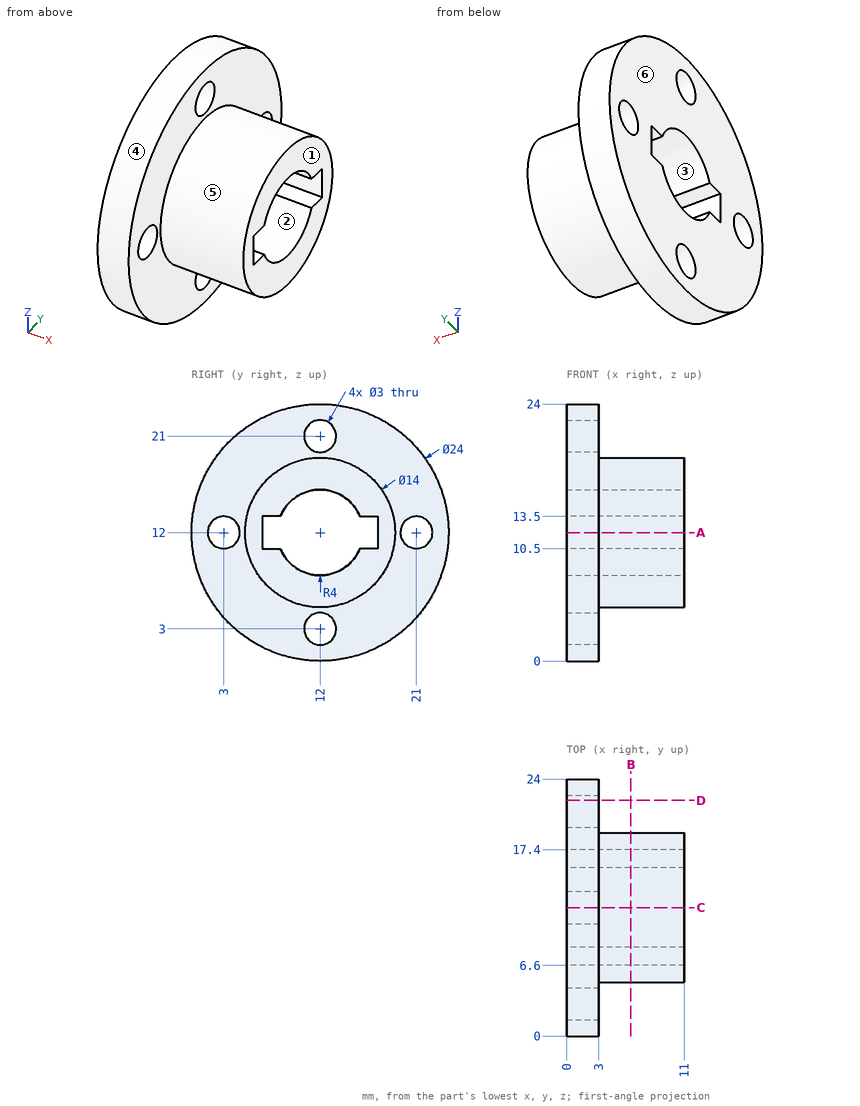
Here's the drawing with two shaded views (mm, measured from the low corner). I have some questions. A direction names the side the tool comes from. Coordinates: 2 decimals unless noted, no trailing zeros. Write each loop counter-clockwise with the first axis right and the second up, starting at its lowest first coordinate (ties: lowest second). Pieces come first, ordered by that corner, then holes. Notation, with made-up numbers: (37, -38) -> (69, -38) arc R26 cw to (69, -12) -> close; hole circle Ø11 at (-40, 7.5). An arc over 180 degrees is marked (long way). One line per question, with ' | ' between items. Start each with the question number.
1. If we section it at D-D (y = 22): Please give me the cut outline in (x, z), and give its area (3 significant figures).
2. Will these pins go through, and if not, where does the flat tip stop? P1, Ø0.5, axis at x = 4, y = 8, coming from the -Z side; P2, Ø1, axis at x = 6, y = 6, coming from the -Z side; P3, Ø3, axis at x = 7, y = 18.5, coming from the +Z side; P4, Ø2.5, axis at y = 12, z = 21, coming from the +X side.
3. Thinking about a two-plate mould opening in Z: for the marked faces 1, 2, 3 and 4, which applies, pulls with the +Z half, pulls with the -Z half, needs draft (parallel to the pull), parting line crosses it, or undercut?
4. If we section it at B-B (x = 6): Please give me the cut outline in (y, z).
5. Please list where these lines run through material, in increasing order: line 1 along Y through (x, z) = (1.7, 12); line 2 along Y through (x, z) = (1.5, 13); line 3 along X through (y, z) = (21.25, 4.5).
6. If we section it at C-C (y = 12): Please give me the cut outline in (x, z), and give its area (3 significant figures).
7. If we section it at A-A (z = 12): Please give me the cut outline in (x, y), and give its area (3 significant figures).
8. For the marked faces 5 and 6, which set-ups out of +Z, -Z, +X, -X, +Y, -Y let a thin tool reach every point of the face, with its end or its side?
Return value:
1) outline: (0, 5.37) -> (3, 5.37) -> (3, 10.88) -> (0, 10.88) -> close; (0, 13.12) -> (3, 13.12) -> (3, 18.63) -> (0, 18.63) -> close | area: 33.1 mm²
2) P1: stops at z = 6.09 | P2: stops at z = 7.67 | P3: stops at z = 16.9 | P4: passes through
3) face 1: needs draft | face 2: undercut | face 3: undercut | face 4: parting line crosses it
4) outline: circle Ø14 at (12, 12); hole (6.6, 10.5) -> (8.29, 10.5) arc R4 ccw to (15.71, 10.5) -> (17.4, 10.5) -> (17.4, 13.5) -> (15.71, 13.5) arc R4 ccw to (8.29, 13.5) -> (6.6, 13.5) -> close
5) line 1: y = 0 to 1.5, 4.5 to 6.6, 17.4 to 19.5, 22.5 to 24 | line 2: y = 0.04 to 1.88, 4.12 to 6.6, 17.4 to 19.88, 22.12 to 23.96 | line 3: x = 0 to 3
6) outline: (0, 0) -> (3, 0) -> (3, 1.5) -> (0, 1.5) -> close; (0, 4.5) -> (3, 4.5) -> (3, 5) -> (11, 5) -> (11, 8) -> (0, 8) -> close; (0, 16) -> (11, 16) -> (11, 19) -> (3, 19) -> (3, 19.5) -> (0, 19.5) -> close; (0, 22.5) -> (3, 22.5) -> (3, 24) -> (0, 24) -> close | area: 78.0 mm²
7) outline: (0, 0) -> (3, 0) -> (3, 1.5) -> (0, 1.5) -> close; (0, 4.5) -> (3, 4.5) -> (3, 5) -> (11, 5) -> (11, 6.6) -> (0, 6.6) -> close; (0, 17.4) -> (11, 17.4) -> (11, 19) -> (3, 19) -> (3, 19.5) -> (0, 19.5) -> close; (0, 22.5) -> (3, 22.5) -> (3, 24) -> (0, 24) -> close | area: 47.2 mm²
8) face 5: +X | face 6: +Z, -Z, -X, +Y, -Y
